Work out the finished part from the listing and answer in its coordinate system (mm). A direction names the side the tool comes from. Round coordinates to 2 decimals unless told otherwise and drop trailing zeros. Write each loop counter-clockwise with the first axis right and the second up, starting at its lowest first coordinate (ties: lowest second). Pieces come first, ordered by that corner, then holes.
1. Find section C-C (y = -3). Write down the section's boundary in (x, z), and give its area (3 significant figures).
2. Find section A-A (x = 1). Write down the section's boundary in (y, z), and give its area (3 significant figures).
3. Find section D-D (z = -9.05). Write down the section's boundary in (x, y) (3 decimals).
4. Find section B-B (y = -16). Write down the section's boundary in (x, z), and give its area (3 significant figures).
5. A tool of negligible diameter and unlimited length cuts with its end or side. For faces 1 (the face through (0.99, 4.88, 1.08)), 2 (the face through (9.51, -1.22, -9.25)), 3 (the face through (1, -12, -13.55)), 4 (the face through (1.225, -3.905, 0.867)), from which of +Z, -Z, +X, -X, +Y, -Y can it reach the whole face along a straight path? Write none if from no direction.
6. Determine the mould class of faces 5 (the face through (-6.8, -6, 0)), 6 (the face through (-7.8, -5, 0)), 7 (the face through (9.51, 9.67, 0.17)) for opening direction X: pulls with the +X half, pulls with the -X half, needs draft (parallel to the pull), parting line crosses it, or undercut.
7. Flat-ended cylindrical pins translate along their axes: pin 1 Ø8 at (x, y) = (-3, 6.5) entering from +Z; pin 2 Ø2 at (y, z) = (0, -9.525) entering from +X; pin 3 Ø1 at (x, y) = (3.5, 1) entering from -Z; pin 4 Ø7 at (y, z) = (0, 0) entering from +X. Find the tip coordinate at first contact, or state that the pin passes through.
8. Straight lines are drawn through the part: probe 1 along Y at (x, z) = (-3, 0); probe 2 along X at (y, z) = (-10, 1.75); probe 3 along Z at (x, y) = (-3.5, -6). For each, find the intervals that lie inside material, in ascending order.
Autodesk Inventor part; units mm, degrees
ref_plane "Arbeitsebene1" through (0, 0, 0) normal (1, 0, 0) x (0, 0, -1)
ref_plane "YZ Plane" through (0, 0, 0) normal (1, 0, 0) x (0, 1, 0)
ref_plane "XZ Plane" through (0, 0, 0) normal (0, 1, 0) x (-1, 0, 0)
ref_plane "Arbeitsebene1" through (0, 0, 0) normal (1, 0, 0) x (0, 0, -1)
sketch "Skizze1" plane through (0, 0, 0) normal (1, 0, 0) x (0, 0, -1)
  arc A0 (14.55, 0) -> (-14.55, 0) centre (0, 0) ccw
  line L0 (14.55, 0) -> (14.55, -25.15)
  line L1 (14.55, -25.15) -> (-14.55, -25.15)
  line L2 (-14.55, -25.15) -> (-14.55, 0)
  circle A1 centre (0, 0) radius 4
  line L3 (-20.37, 0) -> (20.37, 0) construction
  line L4 (0, -33.09) -> (0, 22.49) construction
  circle A2 centre (0, 10.45) radius 0.8
  circle A3 centre (9.525, 0) radius 1.25
  circle A4 centre (-9.525, 0) radius 1.25
  circle A5 centre (-9.05, -5.225) radius 0.8
  circle A6 centre (9.05, -5.225) radius 0.8
  circle A7 centre (0, 0) radius 10.45 construction
  line L5 (0, 0) -> (9.05, -5.225) construction
  line L6 (0, 0) -> (-9.05, -5.225) construction
  circle A8 centre (0, 0) radius 9.525 construction
  point P0 (0, 14.55)
  dimension "d0" = 29.1
  dimension "d1" = 39.7
  dimension "d2" = 8
  dimension "d9" = 1.6
  dimension "d11" = 120
  dimension "d12" = 20.9
  dimension "d13" = 2.5
  dimension "d14" = 19.05
extrude "Extrusion1" add sketch "Skizze1" along normal blind 10 and the other way blind 7.8 contours L0 L1 L2 A0 | A2 | A3 | A4 | A5 | A6
shell "Wandung1" thickness 1 removed faces 1 at (4.0667, -25.15, -4.85)
extrude "Extrusion2" cut sketch "Skizze1" against normal blind 10 from surface at 10 contours A2 | A3 | A4 | A5 | A6
properties part number "EncoderEnclosure"
Worked answers:
1. outline: (-7.8, -14.55) - (10, -14.55) - (10, -2.65) - (-7.8, -2.65) - close; (-7.8, 2.65) - (10, 2.65) - (10, 14.55) - (-7.8, 14.55) - close; hole (-6.8, -13.55) - (9, -13.55) - (9, -4) - (-6.8, -4) - close; hole (-6.8, 4) - (9, 4) - (9, 13.55) - (-6.8, 13.55) - close
1. area: 122 mm2
2. outline: (-25.15, -14.55) - (0, -14.55) arc R14.55 ccw to (0, 14.55) - (-25.15, 14.55) - (-25.15, 13.55) - (0, 13.55) arc R13.55 cw to (0, -13.55) - (-25.15, -13.55) - close; circle Ø10 at (0, 0); hole circle Ø8 at (0, 0)
2. area: 123 mm2
3. outline: (-7.8, -25.15) - (-6.8, -25.15) - (-6.8, 10.085) - (9, 10.085) - (9, 1.156) - (10, 1.156) - (10, 11.393) - (-7.8, 11.393) - close; (9, -25.15) - (10, -25.15) - (10, -6.025) - (9, -6.025) - close; (9, -4.425) - (10, -4.425) - (10, -1.156) - (9, -1.156) - close
4. outline: (-7.8, -14.55) - (10, -14.55) - (10, 14.55) - (-7.8, 14.55) - close; hole (-6.8, -13.55) - (9, -13.55) - (9, 13.55) - (-6.8, 13.55) - close
4. area: 89.8 mm2
5. face 1: none
5. face 2: +X
5. face 3: -Y
5. face 4: +X, -X
6. face 5: undercut
6. face 6: pulls with the -X half
6. face 7: needs draft
7. pin 1: stops at z = 14.33
7. pin 2: stops at x = -6.8
7. pin 3: stops at z = -14.54
7. pin 4: passes through
8. probe 1: y = -5 to -4, 4 to 5, 13.55 to 14.55
8. probe 2: x = -7.8 to -6.8, 9 to 10
8. probe 3: z = -14.55 to -13.55, 13.55 to 14.55
